Drawing for the job (mm, zero at the part's lowest x, y, z). A direction names the side the tool comes from. Give positions to 0.01 mm unless a question says otherwise; leave off trailing zeros. Write each loop counter-clockwise with the first axis right and the second up, starting at its lowest first coordinate (ties: lowest second). Pieces come first, ordered by that corner, then holes.
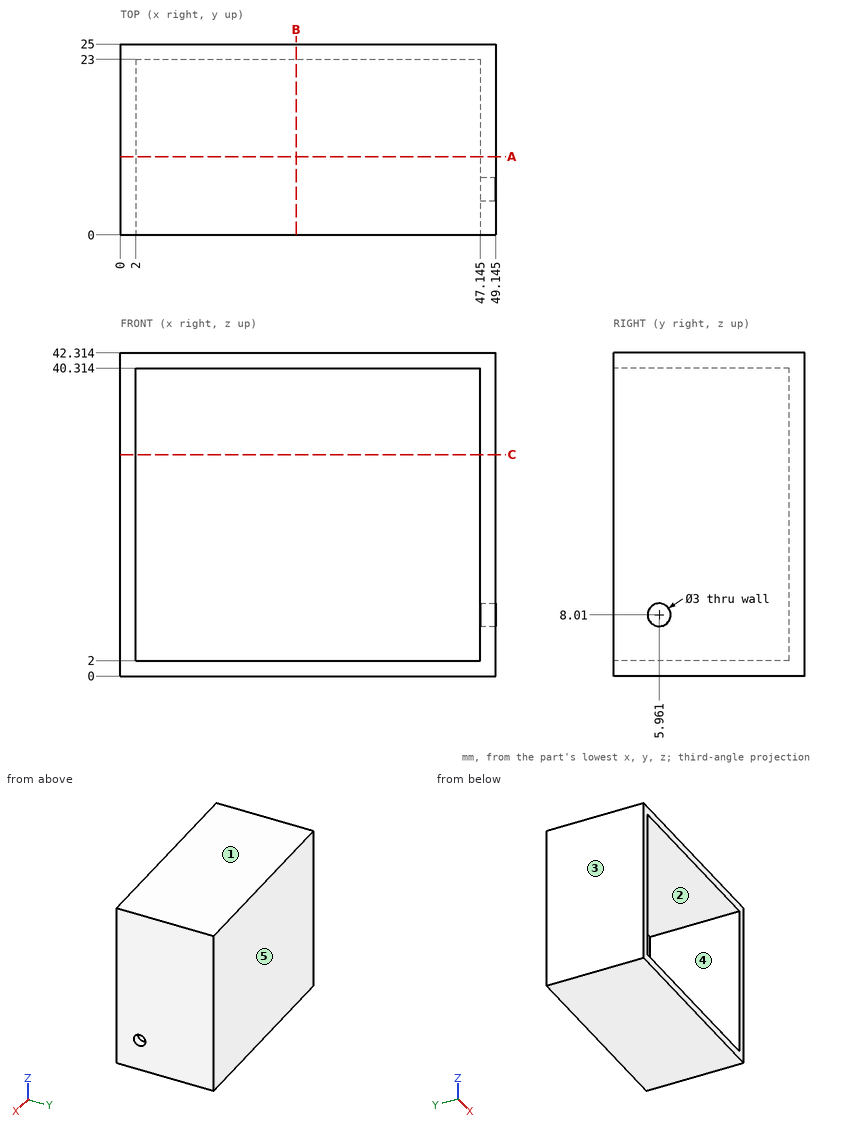
1. Which spindle directions (+Z, -Z, +X, -X, +Y, -Y) get a long thin tool onto all of the face, cutting with end or side? Do the marked faces 1 and 2. Say none if no direction does.
Calculated:
face 1: +Z, +X, -X, +Y, -Y
face 2: -Y
2. Slice it at C-C, the plane z = 29. Write the cut outline in (x, y) (1 decimal).
Calculated:
outline: (0, 0) - (2, 0) - (2, 23) - (47.1, 23) - (47.1, 0) - (49.1, 0) - (49.1, 25) - (0, 25) - close
3. Probe probe 1 along Z at (x, y) = (3, 7.5); probe 2 along X at (y, z) = (8.75, 33.5) (1 decimal); probe 3 along Y at (x, z) = (43, 25). List the from-to ranges inside material, lowest first.
Calculated:
probe 1: z = 0 to 2, 40.31 to 42.31
probe 2: x = 0 to 2, 47.1 to 49.1
probe 3: y = 23 to 25
4. Pin check, flat tips, straight feed: P1, Ø10, axis at x = 36, y = 9.5, coming from the -Z side; P2, Ø12, axis at x = 19.5, z = 26.5, coming from the -Y side. Stop position of each tip, or through.
Calculated:
P1: stops at z = 0
P2: stops at y = 23
5. Slice it at A-A, the plane y = 10.25. Write the cut outline in (x, z) (1 decimal), and give its area (3 significant figures).
Calculated:
outline: (0, 0) - (49.1, 0) - (49.1, 42.3) - (0, 42.3) - close; hole (2, 2) - (47.1, 2) - (47.1, 40.3) - (2, 40.3) - close
area: 350 mm2
6. Pull direction X, two halves, no side cores. Call the marked faces 3, 4 and 5: +X half, -X half, draft (parallel to the pull), parting line (faces both ways), or undercut.
Calculated:
face 3: -X half
face 4: undercut
face 5: draft
7. Slice it at B-B, the plane x = 23. Write the cut outline in (y, z).
Calculated:
outline: (0, 0) - (25, 0) - (25, 42.31) - (0, 42.31) - (0, 40.31) - (23, 40.31) - (23, 2) - (0, 2) - close
